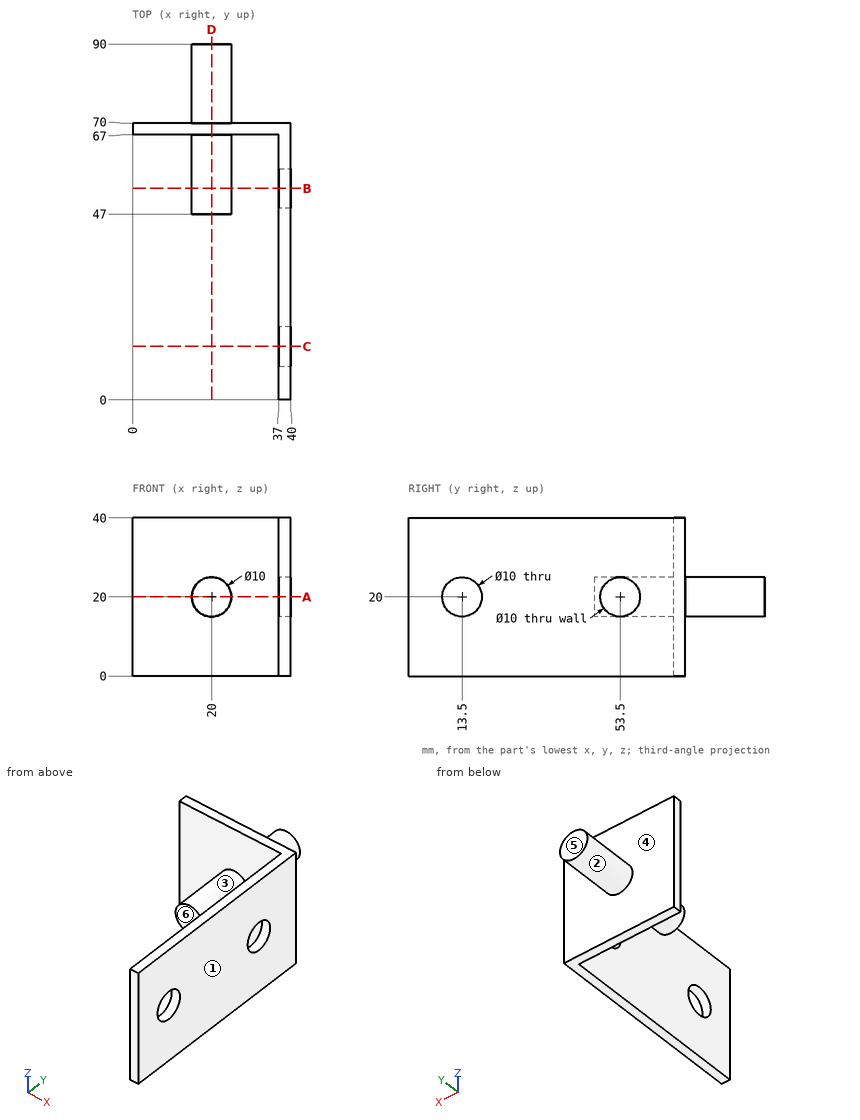
Geometry: see drawing. Coordinates: mm, zero at the bounding-box minimum. A direction names the side the tool comes from. Round coordinates to 2 decimals unless told otherwise and drop trailing zeros. Write each loop counter-clockwise with the first axis right and the second up, starting at its lowest first coordinate (ties: lowest second). Pieces come first, ordered by that corner, then holes.
Item 1: Set-up query: the marked faces 5 and 6. Return all of +Z, -Z, +X, -X, +Y, -Y with unobstructed straight access to the full face (end or side cutting, diameter ignored); none if empty.
Item 2: Mould query, pull axis X, two halves, no side actions, for the marked faces 1, 2, 3 and 4. Classes: +X half, -X half, draft (parallel to the pull), parting line (faces both ways), or undercut.
Item 3: Section query D-D (x = 20). Return loops of the section in (y, z), plus the area to 3 significant figures.
Item 4: Section query C-C (y = 13.5). Return loops of the section in (x, z).
Item 5: Pin query (flat end, axial travel): P1, Ø4, axis at x = 11.5, z = 34, coming from the -Y side; P2, Ø12, axis at x = 29, y = 17.5, coming from the -Z side; P3, Ø8, axis at y = 73, z = 34, coming from the -X side; P4, Ø3, axis at x = 19.5, z = 21, coming from the -Y side. Return the tip coordinate at first contact, or that it passes through.
Item 6: Material intervals for L1, parallel to Z at x = 38.8, y = 53.5; L2, parallel to Y at x = 28, z = 14.5; L3, parallel to X at y = 31, z = 18, sorted ascending.
Item 7: Section query B-B (y = 53.5). Return loops of the section in (x, z).
Item 8: Section query A-A (z = 20). Return loops of the section in (x, y).
Completed:
1. face 5: +Z, -Z, +X, -X, +Y
1. face 6: +Z, -Z, -X, -Y
2. face 1: +X half
2. face 2: parting line
2. face 3: undercut
2. face 4: draft
3. outline: (47, 15) - (67, 15) - (67, 0) - (70, 0) - (70, 15) - (90, 15) - (90, 25) - (70, 25) - (70, 40) - (67, 40) - (67, 25) - (47, 25) - close
3. area: 520 mm2
4. outline: (37, 0) - (40, 0) - (40, 15) - (37, 15) - close; (37, 25) - (40, 25) - (40, 40) - (37, 40) - close
5. P1: stops at y = 67
5. P2: passes through
5. P3: stops at x = 0
5. P4: stops at y = 47
6. L1: z = 0 to 15, 25 to 40
6. L2: y = 67 to 70
6. L3: x = 37 to 40
7. outline: circle Ø10 at (20, 20); (37, 0) - (40, 0) - (40, 15) - (37, 15) - close; (37, 25) - (40, 25) - (40, 40) - (37, 40) - close
8. outline: (0, 67) - (15, 67) - (15, 47) - (25, 47) - (25, 67) - (37, 67) - (37, 58.5) - (40, 58.5) - (40, 70) - (25, 70) - (25, 90) - (15, 90) - (15, 70) - (0, 70) - close; (37, 0) - (40, 0) - (40, 8.5) - (37, 8.5) - close; (37, 18.5) - (40, 18.5) - (40, 48.5) - (37, 48.5) - close
